Source: CAD feature listing. Evaluate the final solid. Frame: model axes, mm. A direction names the side the tool comes from. Round coordinates to 2 decimals unless told otherwise and drop trailing zeros. Loops run counter-clockwise (first coordinate to the right, second up) from the corner with the lowest first, then second, coordinate; pieces in that order, holes last. Notation, with made-up numbers: (33, 3) -> (72, 3) arc R18 ccw to (72, 9) -> close; hole circle Ø7 at (-21, 8.5). An arc over 180 degrees is marked (long way). Write item = value, one per line.
from build123d import *

# Parameters (mm, degrees)
SKETCH1_W           = 67
SKETCH1_H           = 55
BOSS_EXTRUDE1_DEPTH = 19
SKETCH3_W           = 13
SKETCH3_H           = 61
CUT_EXTRUDE1_DEPTH  = 51
FILLET1_R           = 4
FILLET2_R           = 3


with BuildPart() as part:
    # Sketch1 → Boss-Extrude1 (new body)
    with BuildSketch(Plane.YZ):
        Rectangle(SKETCH1_W, SKETCH1_H)
    extrude(amount=BOSS_EXTRUDE1_DEPTH)

    # Sketch3 → Cut-Extrude1 (cut)
    with BuildSketch(Plane.XY.offset(27.5)):
        with Locations((9.5, 0)):
            Rectangle(SKETCH3_W, SKETCH3_H)
    extrude(amount=-CUT_EXTRUDE1_DEPTH, mode=Mode.SUBTRACT)

    # Fillet1
    fillet1_edges = [part.edges().sort_by_distance(p)[0] for p in [
        (19, -33.5, 0),
        (19, 33.5, 0),
    ]]
    fillet(fillet1_edges, radius=FILLET1_R)

    # Fillet2
    fillet2_edges = [part.edges().sort_by_distance(p)[0] for p in [
        (16, 30.5, 2),
        (16, -30.5, 2),
    ]]
    fillet(fillet2_edges, radius=FILLET2_R)


solid = part.part
1. Section query B-B (y = -13). Return the cut outline in (x, z).
Evaluation:
outline = (0, -27.5) -> (19, -27.5) -> (19, 27.5) -> (16, 27.5) -> (16, -23.5) -> (3, -23.5) -> (3, 27.5) -> (0, 27.5) -> close
2. Contact query for flat-ended pins moving along their axis: pin 1 Ø3 at (y, z) = (-20.5, 15.5) entering from -X; pin 2 Ø10 at (x, y) = (10, 13.5) entering from +Z. Output: stop coordinate, or through.
Evaluation:
pin_1 = 0
pin_2 = -23.5
3. Mould query, pull axis Y, two halves, no side actions, for faces 1 (the face through (0, 0, 0)), 2 (the face through (16, 0, 2)), 3 (the face through (17.797, -32.359, 0.385)). Classes: released by +Y, released by -Y, zero draft, split by the parting line, or undercut.
Evaluation:
face_1 = zero draft
face_2 = undercut
face_3 = released by -Y
4. Section query C-C (x = 11). Return the cut outline in (y, z).
Evaluation:
outline = (-33.5, -27.5) -> (33.5, -27.5) -> (33.5, 27.5) -> (30.5, 27.5) -> (30.5, -23.5) -> (-30.5, -23.5) -> (-30.5, 27.5) -> (-33.5, 27.5) -> close
5. Line query: probe 1 along X at (y, z) = (-9.5, 8); probe 2 along Y at (x, z) = (7.75, 5.5); probe 3 along Z at (x, y) = (11.5, 17.5). Output: solid intervals per line, ascending. Write a range as from..to.
Evaluation:
probe_1 = 0..3, 16..19
probe_2 = -33.5..-30.5, 30.5..33.5
probe_3 = -27.5..-23.5
6. Set-up query: faces 4 (the face through (9, 0, -27.5)), 5 (the face through (8, 30.5, 2)). Return all of +Z, -Z, +X, -X, +Y, -Y with unobstructed straight access to the full face (end or side cutting, diameter ignored); none if empty.
Evaluation:
face_4 = -Z, +X, -X, +Y, -Y
face_5 = +Z
7. Section query A-A (z = -6). Return the cut outline in (x, y), then the cut area to 3 significant figures.
Evaluation:
outline = (0, -33.5) -> (15, -33.5) arc R4 ccw to (19, -29.5) -> (19, 29.5) arc R4 ccw to (15, 33.5) -> (0, 33.5) -> close; hole (3, -30.5) -> (13, -30.5) arc R3 ccw to (16, -27.5) -> (16, 27.5) arc R3 ccw to (13, 30.5) -> (3, 30.5) -> close
area = 477 mm²
